The model under review builds one solid part; all positions refer to its coordinate system, in mm. Face numbers are marked on the shaded views. A direction names the side the tool comes from. Round coordinates to 2 decimals unless told otherwise and drop trailing zeros. Write each loop counter-clockwise with the first axis right and the second up, starting at its lowest first coordinate (ties: lowest second). Pieces come first, ordered by that corner, then holes. Notation, with made-up numbers: (-8.75, -7.75) -> (28.25, -7.75) arc R36 cw to (28.25, 31.25) -> close; hole circle Ø2 at (58, 64.5). An arc over 180 degrees is marked (long way). Answer as a JSON object with one key per item and string values. Group by question number.
1) Machinability: for the marked faces 1, 2, 3, 4 and 5, which of the approach directions +Z, -Z, +X, -X, +Y, -Y give a long, thin tool a straight path to every point of the face, cutting with its end or side? Answer none if there is none.
2) Mouldability with a two-part tool opening along Y and no side actions: class the marked faces 6, 7 and 8 as pulls with the +Y half, pulls with the -Y half, needs draft (parallel to the pull), parting line crosses it, or undercut.
3) To check wall thickness, follow probe 1 along X at (y, z) = (-45, -23.5); probe 2 along Z at (x, y) = (0, -3); probe 3 along Z at (x, y) = (0, 7.25). State the ranges of each line that lie inside material, in increasing order. Write a range as [from, to].
4) We need section B-B, the plane z = 10.5. Write out the cut boundary in (x, y) (3 decimals).
5) We need section C-C, the plane z = -20. Write out the cut boundary in (x, y), then the cut area to 3 significant figures.
6) We need section D-D, the plane y = -26. Write out the cut boundary in (x, z), then the cut area to 3 significant figures.
7) We need section A-A, the plane x = 0. Write out the cut boundary in (y, z) (3 decimals).
8) Insertion check: pin 1 Ø6.5 at (x, z) = (0.5, 15.5) entering from -Y; pin 2 Ø12 at (x, y) = (-46, -10.5) entering from -Z; pin 3 Ø5 at (x, y) = (15, -14) entering from -Z; pin 4 Ø1.5 at (x, y) = (-19.5, -67) entering from +Z. Each pin has a flat end and moves straight along its axis. Give the tip position at first contact, or say it passes through.
from build123d import *

# Parameters (mm, degrees)
F0_R      = 3.175
F1_DEPTH  = 6.35
F2_DEPTH  = 6.35
F3_DEPTH  = 9.525
F4_W      = 12.7
F4_H      = 6.35
F5_DEPTH  = 19.05
F6_DEPTH  = 25.4
F7_W      = 127
F7_H      = 12.7
F8_DEPTH  = 76.2
F9_W      = 114.3
F9_H      = 69.85
F10_DEPTH = 10.16


with BuildPart() as f1:
    # F0 (on Front) → F1 (new body)
    with BuildSketch(Plane.XZ):
        Polygon((6.288046, 27.041709), (0, 27.041709), (-6.411954, 27.041709), (-6.411954, -14.614291), (-63.561954, -14.614291), (-63.561954, -27.314291), (-6.411954, -27.314291), (6.288046, -27.314291), (63.438046, -27.314291), (63.438046, -14.614291), (6.288046, -14.614291), align=None)
        with Locations((0, 15.235816)):
            Circle(F0_R, mode=Mode.SUBTRACT)
    extrude(amount=F1_DEPTH)

    # F0 (on Front) → F2 (join)
    with BuildSketch(Plane.XZ):
        Polygon((-6.411954, 27.041709), (0, 27.041709), (6.288046, 27.041709), (6.288046, 31.804209), (-6.411954, 31.804209), align=None)
    extrude(amount=F2_DEPTH)

    # F0 (on Front) → F3 (join)
    with BuildSketch(Plane.XZ):
        Polygon((-6.411954, 27.041709), (0, 27.041709), (6.288046, 27.041709), (6.288046, 31.804209), (-6.411954, 31.804209), align=None)
    extrude(amount=-F3_DEPTH)

    # F4 (on face) → F5 (join)
    with BuildSketch(Plane(origin=(0, 0, 27.041709), x_dir=(1, 0, 0), z_dir=(0, 0, -1))):
        with Locations((-0.061954, -6.35)):
            Rectangle(F4_W, F4_H)
    extrude(amount=F5_DEPTH)

    # F0 (on Front) → F6 (cut)
    with BuildSketch(Plane.XZ):
        with Locations((0, 15.235816)):
            Circle(F0_R)
    extrude(amount=-F6_DEPTH, mode=Mode.SUBTRACT)

    # F7 (on face) → F8 (join)
    with BuildSketch(Plane.XZ.offset(6.35)):
        with Locations((-0.061954, -20.964291)):
            Rectangle(F7_W, F7_H)
    extrude(amount=F8_DEPTH)

    # F9 (on face) → F10 (cut)
    with BuildSketch(Plane(origin=(0, 0, -27.314291), x_dir=(1, 0, 0), z_dir=(0, 0, -1))):
        with Locations((-0.061954, 41.275)):
            Rectangle(F9_W, F9_H)
    extrude(amount=-F10_DEPTH, mode=Mode.SUBTRACT)


solid = f1.part
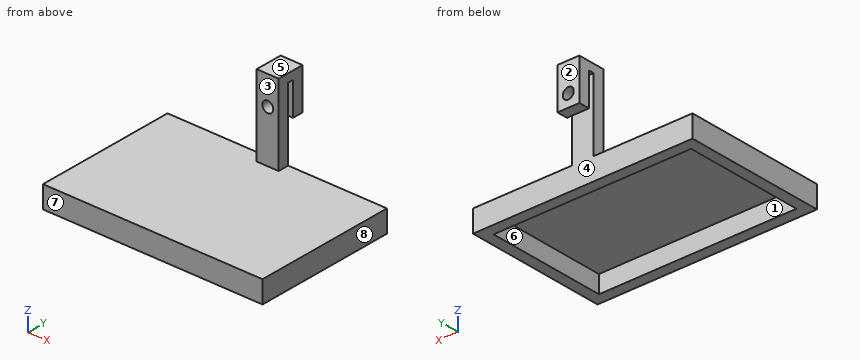
Here are the results:
{
 "1": {"face 1": "-Z", "face 2": "+Z, -Z, +X, -X, +Y", "face 3": "+Z, +X, -X, -Y", "face 4": "-Z, +X, -X", "face 5": "+Z, +X, -X, +Y, -Y"},
 "2": {"face 6": "undercut", "face 7": "pulls with the -Y half", "face 8": "needs draft"},
 "3": {"probe 1": "x = [-63.56, -57.21], [57.09, 63.44]", "probe 2": "z = [-27.31, 12.06], [18.41, 31.8]", "probe 3": "z = [7.99, 12.06], [18.41, 31.8]"},
 "4": {"outline": "(-6.412, -6.35) -> (6.288, -6.35) -> (6.288, 0) -> (-6.412, 0) -> close; (-6.412, 3.175) -> (6.288, 3.175) -> (6.288, 9.525) -> (-6.412, 9.525) -> close"},
 "5": {"outline": "(-63.56, -82.55) -> (63.44, -82.55) -> (63.44, 0) -> (-63.56, 0) -> close; hole (-57.21, -76.2) -> (57.09, -76.2) -> (57.09, -6.35) -> (-57.21, -6.35) -> close", "area": "2,500 mm^2"},
 "6": {"outline": "(-63.56, -27.31) -> (-57.21, -27.31) -> (-57.21, -17.15) -> (57.09, -17.15) -> (57.09, -27.31) -> (63.44, -27.31) -> (63.44, -14.61) -> (-63.56, -14.61) -> close", "area": "452 mm^2"},
 "7": {"outline": "(-82.55, -27.314) -> (-76.2, -27.314) -> (-76.2, -17.154) -> (-6.35, -17.154) -> (-6.35, -27.314) -> (0, -27.314) -> (0, 12.061) -> (-6.35, 12.061) -> (-6.35, -14.614) -> (-82.55, -14.614) -> close; (-6.35, 18.411) -> (0, 18.411) -> (0, 27.042) -> (3.175, 27.042) -> (3.175, 18.411) -> (9.525, 18.411) -> (9.525, 31.804) -> (-6.35, 31.804) -> close; (3.175, 7.992) -> (9.525, 7.992) -> (9.525, 12.061) -> (3.175, 12.061) -> close"},
 "8": {"pin 1": "stops at y = -6.35", "pin 2": "stops at z = -27.31", "pin 3": "stops at z = -17.15", "pin 4": "stops at z = -14.61"}
}
